Design review of the part built by this model. Coordinates are the model's own, in mm. A direction names the side the tool comes from. Coordinates: 2 decimals unless noted, no trailing zeros. Loops run counter-clockwise (first coordinate to the right, second up) from the corner with the lowest first, then second, coordinate; pieces in that order, holes last. Notation, with made-up numbers: (38.25, -15.5) - (55.25, -15.5) arc R21 cw to (55.25, 18.5) - close; hole circle Ø8 at (47.5, 36). An arc over 180 degrees is marked (long way). Use one line per item in the form item = value. Start each with the question number.
(1) Add section C-C (x = 4). State the section outline as (y, z) points, plus the area to 3 significant figures.
(2) Tool access review of faces 1 (the face through (0, -22, 2)), 2 (the face through (12, -17, 2)), 3 (the face through (4, -5, 1)), 4 (the face through (12, -9, 2)), 5 (the face through (-5, -15, 3)): name each direction out of +Z, -Z, +X, -X, +Y, -Y from which nothing blocks a thin tool from reaching the whole face with its end or side.
(3) Add section D-D (y = -13). State the section outline as (x, z) points.
(4) Clearance check with flat-ended pins moving along their axes: pin 1 Ø2 at (y, z) = (-3.5, 1.5) entering from +X; pin 2 Ø2 at (x, z) = (-4.5, 2) entering from +Y; pin 3 Ø1.2 at (x, z) = (-3.5, 1.5) entering from -Y. State where each tip first meets the part, or that it passes through.
(5) For L1, parallel to Y at x = 4, z = 0.65; L2, parallel to Y at x = 4, z = 3.1; L3, parallel to Y at x = -2.75, z = 1.15, list the stretches that pass through material, from the lowest coordinate up.
(6) Add section A-A (x = -5). State the section outline as (y, z) points.
(7) Add section B-B (y = -3). State the section outline as (x, z) points, plus the area to 3 significant figures.
(8) The part is to be moulded in two halves that separate along Y. For faces 6 (the face through (4.354, -24.593, 0.493)), 7 (the face through (-3.443, -12.51, 3.507)), 8 (the face through (-4, -9, 2)), 9 (the face through (-8, -13, 2)), say which applies: pulls with the +Y half, pulls with the -Y half, needs draft (parallel to the pull), parting line crosses it, or undercut.
```python
from build123d import *

# Parameters (mm, degrees)
SKETCH3_W                                      = 8
SKETCH3_H                                      = 26
SKETCH3_R                                      = 1
SKETCH3_W_2                                    = 24
SKETCH3_H_2                                    = 8
BOSS_EXTRUDE1_DEPTH                            = 4
CBORE_FOR_4_SOCKET_HEAD_CAP_SCREW2_D           = 3.2639
CBORE_FOR_4_SOCKET_HEAD_CAP_SCREW2_CBORE_D     = 5.55752
CBORE_FOR_4_SOCKET_HEAD_CAP_SCREW2_CBORE_DEPTH = 3.000000096
CBORE_FOR_4_SOCKET_HEAD_CAP_SCREW3_D           = 3.2639
CBORE_FOR_4_SOCKET_HEAD_CAP_SCREW3_CBORE_D     = 5.55752
CBORE_FOR_4_SOCKET_HEAD_CAP_SCREW3_CBORE_DEPTH = 3.000000096


with BuildPart() as part:
    # Sketch3 → Boss-Extrude1 (new body)
    # profile 1 of 2: a face of its own
    with BuildSketch(Plane.XY):
        with Locations((4, -13)):
            Rectangle(SKETCH3_W, SKETCH3_H)
        with Locations((4, -3)):
            Circle(SKETCH3_R, mode=Mode.SUBTRACT)
        with Locations((4, -23)):
            Circle(SKETCH3_R, mode=Mode.SUBTRACT)
    # profile 2 of 2: a face of its own
    with BuildSketch(Plane.XY):
        with Locations((4, -13)):
            Rectangle(SKETCH3_W_2, SKETCH3_H_2)
        with Locations((-5, -13)):
            Circle(SKETCH3_R, mode=Mode.SUBTRACT)
        with Locations((13, -13)):
            Circle(SKETCH3_R, mode=Mode.SUBTRACT)
    extrude(amount=BOSS_EXTRUDE1_DEPTH)

    # CBORE for #4 Socket Head Cap Screw2 (through all)
    with Locations(Plane(origin=(4, -3, 4), x_dir=(1, 0, 0), z_dir=(0, 0, 1))):
        with Locations((0, 0), (0, -20)):
            CounterBoreHole(CBORE_FOR_4_SOCKET_HEAD_CAP_SCREW2_D / 2, CBORE_FOR_4_SOCKET_HEAD_CAP_SCREW2_CBORE_D / 2, CBORE_FOR_4_SOCKET_HEAD_CAP_SCREW2_CBORE_DEPTH)

    # CBORE for #4 Socket Head Cap Screw3 (through all)
    with Locations(Plane(origin=(13, -13, 0), x_dir=(-1, 0, 0), z_dir=(0, 0, -1))):
        with Locations((0, 0), (18, 0)):
            CounterBoreHole(CBORE_FOR_4_SOCKET_HEAD_CAP_SCREW3_D / 2, CBORE_FOR_4_SOCKET_HEAD_CAP_SCREW3_CBORE_D / 2, CBORE_FOR_4_SOCKET_HEAD_CAP_SCREW3_CBORE_DEPTH)


solid = part.part
```
Computed values:
q1.outline = (-26, 0) - (-24.63, 0) - (-24.63, 1) - (-25.78, 1) - (-25.78, 4) - (-26, 4) - close; (-21.37, 0) - (-4.63, 0) - (-4.63, 1) - (-5.78, 1) - (-5.78, 4) - (-20.22, 4) - (-20.22, 1) - (-21.37, 1) - close; (-1.37, 0) - (0, 0) - (0, 4) - (-0.22, 4) - (-0.22, 1) - (-1.37, 1) - close
q1.area = 64.1 mm^2
q2.face_1 = +Z, -Z, -X, -Y
q2.face_2 = +Z, -Z, +X, -Y
q2.face_3 = +Z
q2.face_4 = +Z, -Z, +X, +Y
q2.face_5 = -Z
q3.outline = (-8, 0) - (-7.78, 0) - (-7.78, 3) - (-6.63, 3) - (-6.63, 4) - (-8, 4) - close; (-3.37, 3) - (-2.22, 3) - (-2.22, 0) - (10.22, 0) - (10.22, 3) - (11.37, 3) - (11.37, 4) - (-3.37, 4) - close; (14.63, 3) - (15.78, 3) - (15.78, 0) - (16, 0) - (16, 4) - (14.63, 4) - close
q4.pin_1 = 8
q4.pin_2 = -9
q4.pin_3 = -17
q5.L1 = -26 to -24.63, -21.37 to -4.63, -1.37 to 0
q5.L2 = -26 to -25.78, -20.22 to -5.78, -0.22 to 0
q5.L3 = -17 to -14.63, -11.37 to -9
q6.outline = (-17, 0) - (-15.78, 0) - (-15.78, 3) - (-14.63, 3) - (-14.63, 4) - (-17, 4) - close; (-11.37, 3) - (-10.22, 3) - (-10.22, 0) - (-9, 0) - (-9, 4) - (-11.37, 4) - close
q7.outline = (0, 0) - (2.37, 0) - (2.37, 1) - (1.22, 1) - (1.22, 4) - (0, 4) - close; (5.63, 0) - (8, 0) - (8, 4) - (6.78, 4) - (6.78, 1) - (5.63, 1) - close
q7.area = 12.1 mm^2
q8.face_6 = undercut
q8.face_7 = undercut
q8.face_8 = pulls with the +Y half
q8.face_9 = needs draft
